Source: CAD feature listing. Evaluate the final solid. Frame: model axes, mm. Give positions to 0.01 mm unless a question says otherwise; leave off trailing zeros. Order: outer loops, then holes, each group sorted by start corner. A loop starts at its lowest first (then second) coordinate and runs counter-clockwise, first axis right, second up. Notation, with made-up numbers: (30, 35.25) - (71, 35.25) arc R22 ccw to (71, 50.25) - close; hole circle Ø4 at (53.25, 23.5). An arc over 180 degrees is marked (long way). Use CSV: the item, a comma, the result in double quotes.
```python
from build123d import *

# Parameters (mm, degrees)
CROQUIS1_R              = 6
SALIENTE_EXTRUIR1_DEPTH = 16


with BuildPart() as part:
    # Croquis1 → Saliente-Extruir1 (new body)
    with BuildSketch(Plane(origin=(0, 0, 0), x_dir=(1, 0, 0), z_dir=(0, 1, 0))):
        with BuildLine():
            ThreePointArc((27.281229681, -8.245271801), (28.193661042, -4.167430508), (28.5, 0))
            ThreePointArc((28.5, 0), (28.193661042, 4.167430508), (27.281229681, 8.245271801))
            ThreePointArc((27.281229681, 8.245271801), (20.784609691, 12), (20.781229681, 19.50360205))
            ThreePointArc((20.781229681, 19.50360205), (14.25, 24.681724008), (6.5, 27.748873851))
            ThreePointArc((6.5, 27.748873851), (0, 24), (-6.5, 27.748873851))
            ThreePointArc((-6.5, 27.748873851), (-14.25, 24.681724008), (-20.781229681, 19.50360205))
            ThreePointArc((-20.781229681, 19.50360205), (-20.033536457, 17.695055573), (-19.778532486, 15.754731247))
            ThreePointArc((-19.778532486, 15.754731247), (-21.975611771, 10.447131827), (-27.281229681, 8.245271801))
            ThreePointArc((-27.281229681, 8.245271801), (-28.5, 0), (-27.281229681, -8.245271801))
            ThreePointArc((-27.281229681, -8.245271801), (-21.975611771, -10.447131827), (-19.778532486, -15.754731247))
            ThreePointArc((-19.778532486, -15.754731247), (-20.033536457, -17.695055573), (-20.781229681, -19.50360205))
            ThreePointArc((-20.781229681, -19.50360205), (-14.25, -24.681724008), (-6.5, -27.748873851))
            ThreePointArc((-6.5, -27.748873851), (0, -24), (6.5, -27.748873851))
            ThreePointArc((6.5, -27.748873851), (14.25, -24.681724008), (20.781229681, -19.50360205))
            ThreePointArc((20.781229681, -19.50360205), (20.784609691, -12), (27.281229681, -8.245271801))
        make_face()
        with Locations(Location((0, 0, 0), (0, 0, 270))):
            Circle(CROQUIS1_R, mode=Mode.SUBTRACT)
    extrude(amount=SALIENTE_EXTRUIR1_DEPTH)


solid = part.part
```
Item 1: Section D-D on x = -18.5. Return the cut outline in (y, z).
Filled in:
outline,"(0, -21.68) - (16, -21.68) - (16, 21.68) - (0, 21.68) - close"
Item 2: Section C-C on z = 3. Return the cut outline in (x, y).
Filled in:
outline,"(-28.34, 0) - (-5.2, 0) - (-5.2, 16) - (-28.34, 16) - close; (5.2, 0) - (28.34, 0) - (28.34, 16) - (5.2, 16) - close"
Item 3: Section A-A on x = 0. Return the cut outline in (y, z), then the cut area to 3 significant figures.
Filled in:
outline,"(0, -24) - (16, -24) - (16, -6) - (0, -6) - close; (0, 6) - (16, 6) - (16, 24) - (0, 24) - close"
area,"576 mm2"
Item 4: First-contact query: pin 1 (2 mm diameter, centred on x = 2, y = 5.5, fed in from +Z); pin 2 (6 mm diameter, centred on x = 1.5, y = 7, fed in from -Z); pin 3 (7 mm diameter, centred on x = 0, z = 0, fed in from +Y); pin 4 (1 mm diameter, centred on y = 2, z = -4, fed in from -X). Flat tips, straight axial feed; report the tip coordinate or a pass-through.
Filled in:
pin 1,"stops at z = 24.63"
pin 2,"stops at z = -25.5"
pin 3,"passes through"
pin 4,"stops at x = -28.28"
Item 5: Section B-B on y = 2.75. Return the cut outline in (x, z).
Filled in:
outline,"(-27.28, -8.25) arc R7.51 cw to (-20.78, -19.5) arc R28.5 ccw to (-6.5, -27.75) arc R7.51 cw to (6.5, -27.75) arc R28.5 ccw to (20.78, -19.5) arc R7.51 cw to (27.28, -8.25) arc R28.5 ccw to (27.28, 8.25) arc R7.51 cw to (20.78, 19.5) arc R28.5 ccw to (6.5, 27.75) arc R7.51 cw to (-6.5, 27.75) arc R28.5 ccw to (-20.78, 19.5) arc R7.51 cw to (-27.28, 8.25) arc R28.5 ccw to start; hole circle Ø12 at (0, 0)"
Item 6: Material intervals for line 1 (X direction, y = 13.25, z = -15.5); line 2 (Z direction, x = -4.5, y = 6.25); line 3 (Z direction, x = 3.5, y = 5.75), sorted ascending. Write a range as from..to.
Filled in:
line 1,"x = -19.78..19.78"
line 2,"z = -25.5..-3.97, 3.97..25.5"
line 3,"z = -24.87..-4.87, 4.87..24.87"
Item 7: Mould query, pull axis Z, two halves, no side actions, for faces 1 (the cylindrical face through (-28.5, 7.9, -0.1)), 2 (the cylindrical face through (1.802, 7.888, 5.723)), 3 (the flat face through (0, 0, -7)), 4 (the cylindrical face through (0, 8, -24)). Classes: released by +Z, released by -Z, zero draft, split by the parting line, or undercut.
Filled in:
face 1,"split by the parting line"
face 2,"undercut"
face 3,"zero draft"
face 4,"released by -Z"
